Could you check a few things on this drawing? It's one solid part, dimensions in mm from its lowest x, y, z. Give positions to 0.01 mm unless a question says otherwise; leave off trailing zeros. Order: outer loops, then holes, each group sorted by start corner. A loop starts at its lowest first (then second) coordinate and runs counter-clockwise, first axis right, second up. Notation, with made-up numbers: (-6, 88.5) -> (52, 88.5) arc R10 cw to (52, 107.5) -> close; hole circle Ø2 at (54, -12). An arc over 180 degrees is marked (long way). Write each question's results on one line, items separated by ' | '. Start each with the question number.
Q1. Imagine slicing it at D-D, the plane y = 34. Please give me the cut outline in (x, z), then the cut area to 3 significant figures.
Q2. Thinking about a two-plate mould opening in Y: for the marked faces 1, 2 and 3, which applies, pulls with the +Y half, pulls with the -Y half, needs draft (parallel to the pull), parting line crosses it, or undercut?
Q3. I'm going to push flat-ended pins straight in: pin 1 (1.3 mm diameter, centred on x = 17, z = 0.5, fed in from -Y); pin 2 (3 mm diameter, centred on x = 56, y = 39.5, fed in from -Z); pin 3 (0.6 mm diameter, centred on x = 17.5, z = 0.5, fed in from +Y); pin 4 (2 mm diameter, centred on x = 36, z = 4.5, fed in from +Y). Where does each tip first touch, or does it pass through?
Q4. Imagine slicing it at A-A, the plane x = 65. Please give me the cut outline in (y, z), then the cut area to 3 significant figures.
Q5. I need wall thicknesses on line 1 along Y through (x, z) = (40, 3.05); line 2 along Z through (x, y) = (38, 37); line 3 along X through (y, z) = (44.5, 5.5). Which ranges of each line are inside material? Lowest first, please. Write a range as [from, to].
Q6. Imagine slicing it at C-C, the plane z = 2.5. Please give me the cut outline in (x, y), then the cut area to 3 significant figures.
Q7. Imagine slicing it at B-B, the plane x = 40. Please give me the cut outline in (y, z), then the cut area to 4 significant figures.
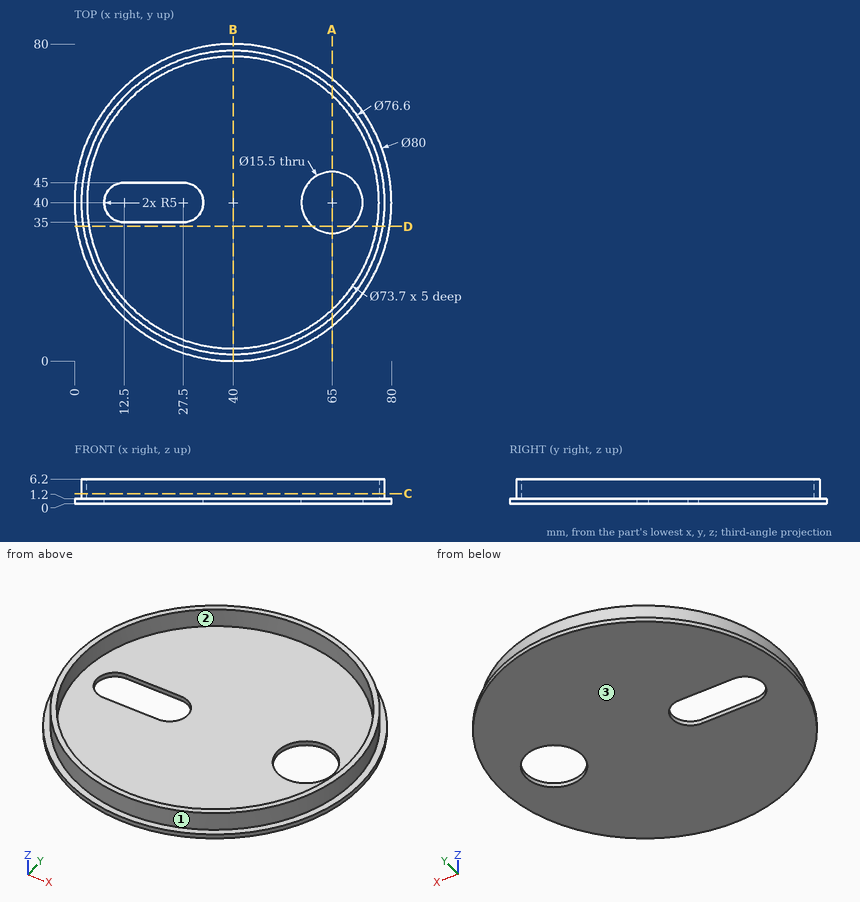
Geometry check:
1) outline: (0.45, 0) -> (60.09, 0) -> (60.09, 1.2) -> (3.64, 1.2) -> (3.64, 6.2) -> (2.17, 6.2) -> (2.17, 1.2) -> (0.45, 1.2) -> close; (69.91, 0) -> (79.55, 0) -> (79.55, 1.2) -> (77.83, 1.2) -> (77.83, 6.2) -> (76.36, 6.2) -> (76.36, 1.2) -> (69.91, 1.2) -> close | area: 97.8 mm²
2) face 1: parting line crosses it | face 2: undercut | face 3: needs draft
3) pin 1: y = 6.83 | pin 2: z = 0 | pin 3: y = 73.27 | pin 4: y = 78.18
4) outline: (8.78, 0) -> (32.25, 0) -> (32.25, 1.2) -> (12.93, 1.2) -> (12.93, 6.2) -> (10.98, 6.2) -> (10.98, 1.2) -> (8.78, 1.2) -> close; (47.75, 0) -> (71.22, 0) -> (71.22, 1.2) -> (69.02, 1.2) -> (69.02, 6.2) -> (67.07, 6.2) -> (67.07, 1.2) -> (47.75, 1.2) -> close | area: 75.8 mm²
5) line 1: [1.7, 3.15], [76.85, 78.3] | line 2: [0, 1.2] | line 3: [1.97, 3.43], [76.57, 78.03]
6) outline: circle Ø76.6 at (40, 40); hole circle Ø73.7 at (40, 40) | area: 342 mm²
7) outline: (0, 0) -> (80, 0) -> (80, 1.2) -> (78.3, 1.2) -> (78.3, 6.2) -> (76.85, 6.2) -> (76.85, 1.2) -> (3.15, 1.2) -> (3.15, 6.2) -> (1.7, 6.2) -> (1.7, 1.2) -> (0, 1.2) -> close | area: 110.5 mm²
